```python
from build123d import *

# Parameters (mm, degrees)
SKETCH1_R                = 4
BOSS_EXTRUDE1_DEPTH      = 110
BOSS_EXTRUDE2_DEPTH      = 8
BOSS_EXTRUDE2_DEPTH_BACK = 8
SKETCH2_R                = 2


with BuildPart() as part:
    # Sketch1 → Boss-Extrude1 (new body)
    with BuildSketch(Plane.XY):
        Circle(SKETCH1_R)
    extrude(amount=BOSS_EXTRUDE1_DEPTH)

    # Sketch2 → Boss-Extrude2 (add, two sides: drawn at the far end of the back side and taken through both)
    with BuildSketch(Plane(origin=(0, 0, 0), x_dir=(1, 0, 0), z_dir=(0, 1, 0)).offset(-BOSS_EXTRUDE2_DEPTH_BACK)):
        with Locations(Location((0, -5, 0), (0, 0, 270))):
            Circle(SKETCH2_R)
    extrude(amount=BOSS_EXTRUDE2_DEPTH + BOSS_EXTRUDE2_DEPTH_BACK)


solid = part.part
```
Read the model definition and answer for the solid it produces. Units are mm, in the model's axes. A direction names the side the tool comes from. Round coordinates to 2 decimals unless told otherwise and drop trailing zeros. Loops run counter-clockwise (first coordinate to the right, second up) from the corner with the lowest first, then second, coordinate; pieces in that order, holes last. Notation, with made-up numbers: (-23.5, -6) -> (32.5, -6) arc R13 ccw to (32.5, 3) -> close; hole circle Ø4 at (-6.5, -3.75). An arc over 180 degrees is marked (long way). One line per item, written item: value.
1) A cutting plane is placed at B-B (z = 5). Determine the outline of the cut face in (x, y).
Answer list:
outline: (-2, -8) -> (2, -8) -> (2, -3.46) arc R4 ccw to (2, 3.46) -> (2, 8) -> (-2, 8) -> (-2, 3.46) arc R4 ccw to (-2, -3.46) -> close
2) Consider L1, parallel to Y at x = 0.25, z = 49.5; L2, parallel to Y at x = 2, z = 56. Determine where each line is inside the solid, lowest interval first. Write a range as [from, to].
Answer list:
L1: y = [-3.99, 3.99]
L2: y = [-3.46, 3.46]
3) Flat-ended cylindrical pins translate along their axes: P1, Ø8, axis at y = 4.5, z = 28, coming from the +X side; P2, Ø1.5, axis at y = 4, z = 74, coming from the -X side; P3, Ø3, axis at x = 0, z = 30.5, coming from the +Y side. Find the tip coordinate at first contact, or state that the pin passes through.
Answer list:
P1: stops at x = 3.97
P2: stops at x = -2.33
P3: stops at y = 4
4) A cutting plane is placed at A-A (x = 0). Determine the outline of the cut face in (y, z).
Answer list:
outline: (-8, 3) -> (-4, 3) -> (-4, 0) -> (4, 0) -> (4, 3) -> (8, 3) -> (8, 7) -> (4, 7) -> (4, 110) -> (-4, 110) -> (-4, 7) -> (-8, 7) -> close
5) For faces 1 (the face through (-0.766, 5.7, 6.847)), 2 (the face through (-0.766, -5.764, 6.847)), 3 (the face through (0, -8, 5)), determine the directions among +Z, -Z, +X, -X, +Y, -Y from which every point of the face is accessible in a straight line to the end or side of a thin tool.
Answer list:
face 1: +Y
face 2: -Y
face 3: +Z, -Z, +X, -X, -Y
6) A cutting plane is placed at D-D (z = 91). Determine the outline of the cut face in (x, y), and give its area (3 significant figures).
Answer list:
outline: circle Ø8 at (0, 0)
area: 50.3 mm²
7) A cutting plane is placed at C-C (y = -5.5). Determine the outline of the cut face in (x, z).
Answer list:
outline: circle Ø4 at (0, 5)
